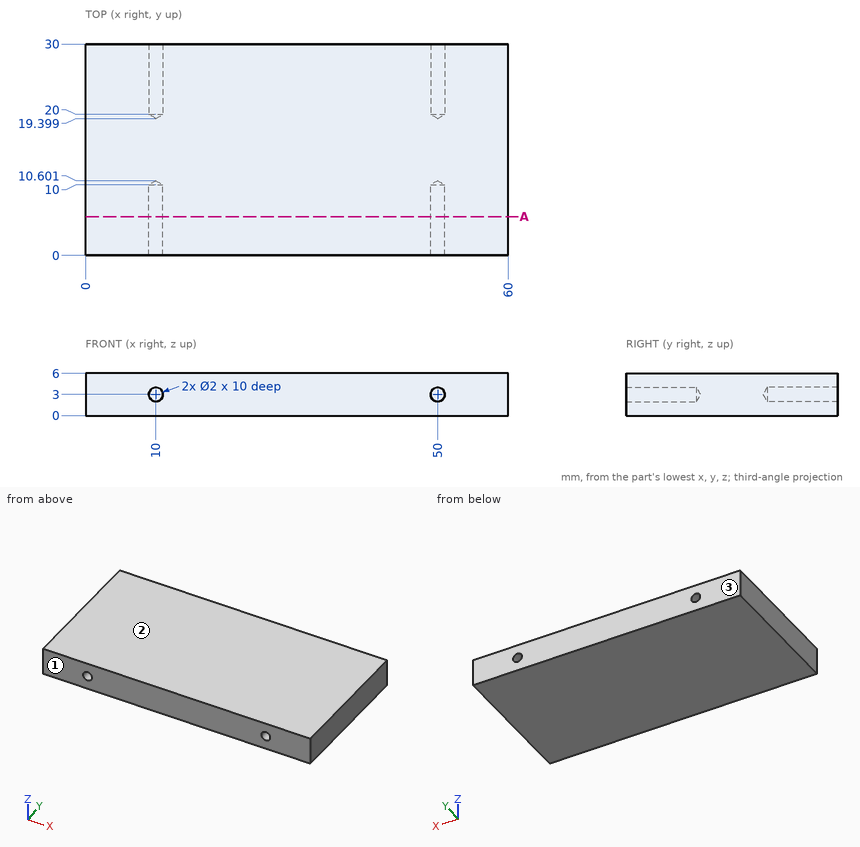
Answer from the drawing. Dimensions are ordinates in mm from the lowest x, y and z of the part. Round coordinates to 2 decimals unless told otherwise and drop trailing zeros. Loops run counter-clockwise (first coordinate to the right, second up) from the corner with the lowest first, then second, coordinate; pieces in that order, holes last.
1) A cutting plane is placed at A-A on y = 5.5. Determine the outline of the cut face in (x, z).
Outcome:
outline: (0, 0) - (60, 0) - (60, 6) - (0, 6) - close; hole circle Ø2 at (10, 3); hole circle Ø2 at (50, 3)
2) For a pull along Y with two mould halves and no side action, classify the marked faces 1, 2 and 3 as released by +Y, released by -Y, zero draft, split by the parting line, or undercut.
Outcome:
face 1: released by -Y
face 2: zero draft
face 3: released by +Y
3) Consider line 1 (X direction, y = 22.5, z = 3); line 2 (Z direction, x = 50, y = 3.5); line 3 (X direction, y = 10.25, z = 2.8). Determine where each line is inside the solid, lowest interval first.
Outcome:
line 1: x = 0 to 9, 11 to 49, 51 to 60
line 2: z = 0 to 2, 4 to 6
line 3: x = 0 to 9.45, 10.55 to 49.45, 50.55 to 60
4) Given P1, Ø1.8, axis at x = 50, z = 3, coming from the +Y side; P2, Ø1.2, axis at x = 50, z = 3, coming from the -Y side; P3, Ø1.8, axis at x = 10, z = 3, coming from the -Y side, each flat-ended and moving along its own axis, determine where each tip first touches the part or whether it passes through.
Outcome:
P1: stops at y = 19.94
P2: stops at y = 10.24
P3: stops at y = 10.06
